Autodesk Inventor part; units mm, degrees
ref_plane "Work Plane1" through (0, 2.5, 0) normal (0, -1, 0) x (1, 0, 0)
ref_plane "YZ Plane" through (0, 0, 0) normal (1, 0, 0) x (0, 1, 0)
ref_plane "XZ Plane" through (0, 0, 0) normal (0, 1, 0) x (-1, 0, 0)
sketch "Sketch1" plane through (0, 0, 0) normal (0, 1, 0) x (-1, 0, 0)
  line L0 (0, 0) -> (59, 0)
  line L1 (59, 0) -> (59, -82)
  line L2 (59, -82) -> (0, -82)
  line L3 (0, -82) -> (0, 0)
  dimension "d0" = 82
  dimension "d1" = 59
extrude "Extrusion1" add sketch "Sketch1" along normal blind 32
ref_plane "Work Plane1" through (0, 2.5, 0) normal (0, -1, 0) x (1, 0, 0)
sketch "Sketch2" plane through (0, 2.5, 0) normal (0, -1, 0) x (1, 0, 0)
  line L0 (-2.5, -2.5) -> (-56.5, -2.5)
  line L1 (-56.5, -2.5) -> (-56.5, -79.5)
  line L2 (-56.5, -79.5) -> (-2.5, -79.5)
  line L3 (-2.5, -79.5) -> (-2.5, -2.5)
  line L4 (0, 0) -> (0, -82)
  line L5 (-59, 0) -> (0, 0)
  line L6 (-59, -82) -> (-59, 0)
  line L7 (0, -82) -> (-59, -82)
  dimension "d5" = 2.5
  dimension "d6" = 2.5
  dimension "d7" = 2.5
  dimension "d8" = 2.5
extrude "Extrusion2" cut sketch "Sketch2" against normal blind 27 contours L3 L2 L1 L0
sketch "Sketch3" plane through (0, 2.5, 0) normal (0, -1, 0) x (1, 0, 0)
  line L0 (-3, -3) -> (-56, -3) construction
  line L1 (-56, -3) -> (-56, -79) construction
  line L2 (-56, -79) -> (-3, -79) construction
  line L3 (-3, -79) -> (-3, -3) construction
  line L4 (-2.5, -2.5) -> (-2.5, -79.5)
  line L5 (-56.5, -2.5) -> (-2.5, -2.5)
  line L6 (-56.5, -79.5) -> (-56.5, -2.5)
  line L7 (-2.5, -79.5) -> (-56.5, -79.5)
  circle A0 centre (-53.8, -24.59) radius 1.65
  circle A1 centre (-5.54, -23.32) radius 1.65
  circle A2 centre (-38.56, -75.39) radius 1.65
  circle A3 centre (-10.62, -75.39) radius 1.65
  point P0 (0, 0)
  dimension "d11" = 0.5
  dimension "d12" = 0.5
  dimension "d13" = 0.5
  dimension "d14" = 0.5
  dimension "d15" = 3.3
  dimension "d16" = 20.32
  dimension "d17" = 2.54
  dimension "d18" = 7.62
  dimension "d19" = 72.39
  dimension "d20" = 21.59
  dimension "d22" = 50.8
  dimension "d23" = 35.56
  dimension "d24" = 72.39
extrude "Extrusion3" cut sketch "Sketch3" along normal blind 27 contours A0 | A1 | A2 | A3
sketch "Sketch4" plane through (-59, 0, 0) normal (0, 0, 1) x (1, 0, 0)
  line L0 (13.4, 5.6) -> (26.4, 5.6)
  line L1 (26.4, 5.6) -> (26.4, 16.5)
  line L2 (26.4, 16.5) -> (13.4, 16.5)
  line L3 (13.4, 16.5) -> (13.4, 5.6)
  line L4 (43.3, 5.6) -> (53.2, 5.6)
  line L5 (53.2, 5.6) -> (53.2, 16.5)
  line L6 (53.2, 16.5) -> (43.3, 16.5)
  line L7 (43.3, 16.5) -> (43.3, 5.6)
  line L8 (56.5, 2.5) -> (2.5, 2.5)
  line L9 (2.5, 2.5) -> (2.5, 29.5)
  line L10 (56.5, 2.5) -> (56.5, 29.5)
  point P0 (59, 0)
  dimension "d27" = 13
  dimension "d28" = 10.9
  dimension "d29" = 9.9
  dimension "d31" = 14
  dimension "d32" = 10.9
  dimension "d33" = 3.3
extrude "Extrusion4" cut sketch "Sketch4" against normal blind 5
sketch "Sketch5" plane through (0, 0, -82) normal (0, 0, -1) x (-1, 0, 0)
  line L0 (11.5, 24.5) -> (33.5, 24.5)
  line L1 (33.5, 24.5) -> (33.5, 20.5)
  line L2 (33.5, 20.5) -> (11.5, 20.5)
  line L3 (11.5, 20.5) -> (11.5, 24.5)
  line L4 (37.5, 24.5) -> (43.5, 24.5)
  line L5 (43.5, 24.5) -> (43.5, 20.5)
  line L6 (43.5, 20.5) -> (37.5, 20.5)
  line L7 (37.5, 20.5) -> (37.5, 24.5)
  line L8 (56.5, 2.5) -> (2.5, 2.5)
  line L9 (2.5, 2.5) -> (2.5, 29.5)
  point P0 (0, 0)
  dimension "d36" = 22
  dimension "d37" = 4
  dimension "d38" = 4
  dimension "d39" = 22
  dimension "d40" = 9
  dimension "d41" = 6
  dimension "d42" = 4
extrude "Extrusion5" cut sketch "Sketch5" against normal blind 5
sketch "Sketch6" plane through (-59, 0, -82) normal (-1, 0, 0) x (0, 0, 1)
  circle A0 centre (57.41, 6) radius 1.6
  line L0 (79.5, 2.5) -> (79.5, 29.5)
  line L1 (82, 0) -> (0, 0)
  dimension "d45" = 3.2
  dimension "d46" = 22.09
  dimension "d47" = 6
sketch "Sketch7" plane through (0, 0, 0) normal (1, 0, 0) x (0, 0, -1)
  circle A0 centre (23.32, 6) radius 1.6
  line L0 (82, 0) -> (0, 0)
  line L1 (2.5, 2.5) -> (2.5, 29.5)
  dimension "d48" = 6
  dimension "d49" = 20.82
  dimension "d50" = 3.2
sketch "Sketch8" plane through (0, 0, -82) normal (0, 0, -1) x (-1, 0, 0)
  circle A0 centre (10.62, 6) radius 1.6
  circle A1 centre (38.56, 6) radius 1.6
  line L0 (59, 0) -> (0, 0)
  line L1 (2.5, 2.5) -> (2.5, 29.5)
  dimension "d51" = 3.2
  dimension "d52" = 3.2
  dimension "d53" = 6
  dimension "d54" = 6
  dimension "d55" = 8.12
  dimension "d56" = 36.06
extrude "Extrusion6" cut sketch "Sketch6" against normal blind 5
extrude "Extrusion7" cut sketch "Sketch7" against normal blind 5
extrude "Extrusion8" cut sketch "Sketch8" against normal blind 5
sketch "Sketch9" plane through (-59, 0, 0) normal (0, 0, 1) x (1, 0, 0)
  line L0 (-2.1645, 16) -> (66.4826, 16)
  line L1 (59, 0) -> (0, 0)
  dimension "d63" = 16
split body "Split1" sketch "Sketch9" result one side removed curves L0 removed pieces at (-39.3333, 31.5, -54.6667)
sketch "Sketch10" plane through (-59, 16, -82) normal (0, 1, 0) x (1, 0, 0)
  line L0 (0, -82) -> (0, 0)
  line L1 (59, 0) -> (59, -82)
  line L2 (0, -82) -> (59, -82)
  line L3 (59, -82) -> (59, 0)
  line L4 (59, 0) -> (0, 0)
  line L5 (0, 0) -> (0, -82)
  line L6 (58, -1) -> (1, -1)
  line L7 (1, -1) -> (1, -81)
  line L8 (1, -81) -> (58, -81)
  line L9 (58, -81) -> (58, -1)
  dimension "d64" = 1
  dimension "d65" = 1
  dimension "d66" = 1
  dimension "d67" = 1
extrude "Extrusion9" add sketch "Sketch10" along normal blind 1
sketch "Sketch11" plane through (-59, 0, 0) normal (0, 0, 1) x (1, 0, 0)
  line L0 (13.4, 16) -> (13.4, 5.6)
  line L1 (58, 17) -> (1, 17)
  line L2 (13.4, 16) -> (26.4, 16)
  line L3 (26.4, 16) -> (26.4, 17)
  line L4 (26.4, 17) -> (13.4, 17)
  line L5 (13.4, 17) -> (13.4, 16)
  line L6 (43.3, 16) -> (43.3, 5.6)
  line L7 (43.3, 16) -> (53.2, 16)
  line L8 (53.2, 16) -> (53.2, 17)
  line L9 (53.2, 17) -> (43.3, 17)
  line L10 (43.3, 17) -> (43.3, 16)
  line L11 (26.4, 16) -> (26.4, 5.6)
  line L12 (53.2, 16) -> (53.2, 5.6)
  point P0 (59, 0)
extrude "Extrusion10" cut sketch "Sketch11" against normal blind 1
properties part number "Arduino_Box_Lower"
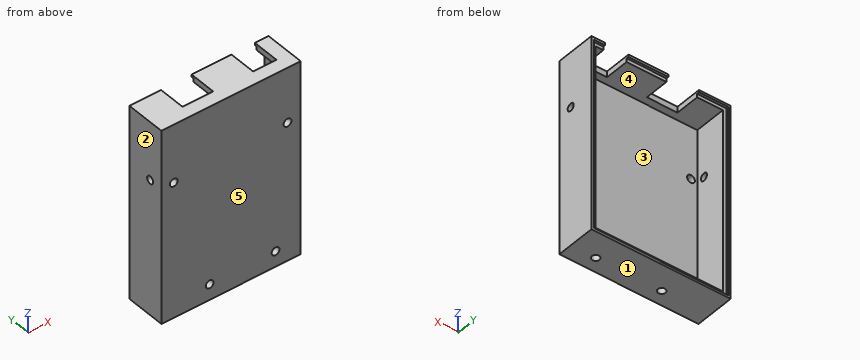
Could you check a few things on this model? Use its own coordinates, in mm. Face numbers are marked on the shaded views. A direction names the side the tool comes from. Give positions to 0.01 mm unless a question says otherwise; leave off trailing zeros. Order: outer loops, then holes, each group sorted by start corner. A loop starts at its lowest first (then second) coordinate and runs counter-clockwise, first axis right, second up.
1. For the marked faces 4 and 5, which set-ups out of +Z, -Z, +X, -X, +Y, -Y let a thin tool reach every point of the face, with its end or its side?
2. Suppose I cut it at D-D (z = -30). List the corners of the cut face in (x, y) for me.
3. We'd pull the mould along Z, two halves only. Please class the marked faces 1, 2 and 3: pulls with the +Z half, pulls with the -Z half, needs draft (parallel to the pull), parting line crosses it, or undercut.
4. Suppose I cut it at C-C (x = -38.56). List the corners of the cut face in (y, z) for me, plus the area to 3 significant figures.
5. Suppose I cut it at A-A (z = -75.39). List the corners of the cut face in (x, y) for me.
6. I need wall thicknesses on L1, parallel to X at y = 0.85, z = -75.39; L2, parallel to Z at x = -35, y = 3; L3, parallel to Y at x = -38.56, z = -80.8. Which ranges of each line are inside material? Lowest first, please.
7. Suppose I cut it at B-B (y = 8.75). List the corners of the cut face in (x, z) for me.
8. Will these pins go through, and if not, where does the flat tip stop? P1, Ø4, axis at x = -20, z = -51.5, coming from the -Y side; P2, Ø3, axis at y = 6, z = -24.59, coming from the -X side; P3, Ø5.5, axis at x = -5.54, z = -23.32, coming from the +Y side; P4, Ø2, axis at x = -13, z = -1.5, coming from the +Y side.
Solved:
1. face 4: +Y
1. face 5: +Z, -Z, +X, -X, -Y
2. outline: (-59, 0) - (0, 0) - (0, 17) - (-1, 17) - (-1, 16) - (-2.5, 16) - (-2.5, 2.5) - (-56.5, 2.5) - (-56.5, 16) - (-58, 16) - (-58, 17) - (-59, 17) - close
3. face 1: pulls with the -Z half
3. face 2: needs draft
3. face 3: undercut
4. outline: (0, -82) - (4.4, -82) - (4.4, -79.5) - (2.5, -79.5) - (2.5, -77.04) - (0, -77.04) - close; (0, -73.74) - (2.5, -73.74) - (2.5, -2.5) - (5.6, -2.5) - (5.6, 0) - (0, 0) - close; (7.6, -82) - (17, -82) - (17, -81) - (16, -81) - (16, -79.5) - (7.6, -79.5) - close
4. area: 231 mm2
5. outline: (-59, 0) - (-40.21, 0) - (-40.21, 2.5) - (-56.5, 2.5) - (-56.5, 16) - (-58, 16) - (-58, 17) - (-59, 17) - close; (-36.91, 0) - (-12.27, 0) - (-12.27, 2.5) - (-36.91, 2.5) - close; (-8.97, 0) - (0, 0) - (0, 17) - (-1, 17) - (-1, 16) - (-2.5, 16) - (-2.5, 2.5) - (-8.97, 2.5) - close
6. L1: x = -59 to -40.21, -36.91 to -12.27, -8.97 to 0
6. L2: z = -82 to -79.5, -2.5 to 0
6. L3: y = 0 to 4.4, 7.6 to 16
7. outline: (-59, -82) - (0, -82) - (0, 0) - (-5.8, 0) - (-5.8, -2.5) - (-2.5, -2.5) - (-2.5, -79.5) - (-56.5, -79.5) - (-56.5, -2.5) - (-45.6, -2.5) - (-45.6, 0) - (-59, 0) - close; (-32.6, -2.5) - (-15.7, -2.5) - (-15.7, 0) - (-32.6, 0) - close
8. P1: stops at y = 0
8. P2: stops at x = -2.5
8. P3: stops at y = 2.5
8. P4: stops at y = 5.6
